Autodesk Inventor part; units mm, degrees
ref_plane "YZ Plane" through (0, 0, 0) normal (1, 0, 0) x (0, 1, 0)
ref_plane "XZ Plane" through (0, 0, 0) normal (0, 1, 0) x (-1, 0, 0)
ref_plane "XY Plane" through (0, 0, 0) normal (0, 0, 1) x (1, 0, 0)
sketch "Sketch1" plane through (0, 0, 0) normal (0, 1, 0) x (-1, 0, 0)
  line L0 (0, 0) -> (180, 0)
  line L1 (180, 0) -> (180, -180)
  line L2 (180, -180) -> (0, -180)
  line L3 (0, -180) -> (0, 0)
  dimension "d0" = 180
  dimension "d1" = 180
extrude "Extrusion1" add sketch "Sketch1" along normal blind 4
chamfer "Chamfer1" distance 2 angle 45 4 edges at (-180, 2, 0) (-180, 2, -180) (0, 2, -180) (0, 2, 0)
sketch "Sketch5" plane through (0, 4, 0) normal (0, 1, 0) x (1, 0, 0)
  line L0 (-165, 165) -> (-15, 165)
  line L1 (-15, 165) -> (-15, 15)
  line L2 (-15, 15) -> (-165, 15)
  line L3 (-165, 15) -> (-165, 165)
  point P0 (0, 0)
  dimension "d29" = 150
  dimension "d30" = 150
  dimension "d31" = 15
  dimension "d32" = 15
extrude "Extrusion5" cut sketch "Sketch5" against normal through all
properties part number "MouldBase20"
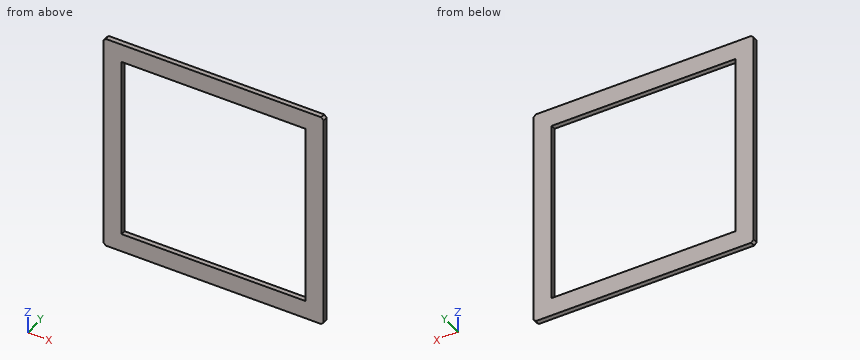
Can you work these out from the model? Positions are in its coordinate system, mm. Coordinates: 2 decimals unless noted, no trailing zeros. Loops run counter-clockwise (first coordinate to the right, second up) from the corner with the lowest first, then second, coordinate; pieces in that order, holes last. Notation, with made-up numbers: (86, 35.5) - (114, 35.5) arc R34 cw to (114, 66.5) - close; hole circle Ø5 at (-32.75, -20.5). An arc over 180 degrees is marked (long way). Use a Markdown table: item, result.
Item 1: I want a section at A-A on x = -61. Please give me the cut outline in (y, z).
Numbers:
| item | result |
|---|---|
| outline | (0, -180) - (4, -180) - (4, -165) - (0, -165) - close; (0, -15) - (4, -15) - (4, 0) - (0, 0) - close |
Item 2: I want a section at B-B on y = 2.05. Please give me the cut outline in (x, z), and give its area (3 significant figures).
Numbers:
| item | result |
|---|---|
| outline | (-180, -178) - (-178, -180) - (-2, -180) - (0, -178) - (0, -2) - (-2, 0) - (-178, 0) - (-180, -2) - close; hole (-165, -165) - (-15, -165) - (-15, -15) - (-165, -15) - close |
| area | 9,890 mm2 |
Item 3: If I drill on probe 1 along Z at (x, y) = (-116, 2.35), over which ranges is the centre line in solid material (lowest first)? Write a range as from..to.
Numbers:
| item | result |
|---|---|
| probe 1 | z = -180..-165, -15..0 |
Item 4: I want a section at C-C on z = -62.5. Please give me the cut outline in (x, y), and give its area (3 significant figures).
Numbers:
| item | result |
|---|---|
| outline | (-180, 0) - (-165, 0) - (-165, 4) - (-180, 4) - close; (-15, 0) - (0, 0) - (0, 4) - (-15, 4) - close |
| area | 120 mm2 |
Item 5: Will this pin go through, and if not, where does the flat tip stop? pin 1 (1.5 mm diameter, centred on x = -105.5, y = 2.5, fed in from +Z).
Numbers:
| item | result |
|---|---|
| pin 1 | stops at z = 0 |
